Geometry check sheet. Reference: the model listing, model coordinates, mm. Face numbers are marked on the shaded views. Coordinates: 2 decimals unless noted, no trailing zeros. Order: outer loops, then holes, each group sorted by start corner. A loop starts at its lowest first (then second) coordinate and runs counter-clockwise, first axis right, second up. Notation, with made-up numbers: (88.5, 50.25) - (96.5, 50.25) arc R8 cw to (96.5, 57.25) - close; hole circle Ø6 at (-10.5, 69.25). An arc over 180 degrees is marked (long way). Return JSON: item names as keys, results as strings. Group by question number.
Item 1: Section check A-A on y = 0. Enter the section's corners in (x, z).
Item 2: Scan lines: probe 1 along Y at (x, z) = (3.8, 0); probe 2 along Z at (x, y) = (3, 2); probe 3 along Y at (x, z) = (4.75, -1). Record each from-to range of solid material in increasing order.
Item 3: Section check C-C on x = 3. Enter the section's corners in (y, z).
Item 4: Draft check along Z on the marked faces 1 and 2. Enter one of: pulls with the +Z half, pulls with the -Z half, needs draft (parallel to the pull), parting line crosses it, or undercut.
Item 5: Gauge pin test, flat ends, axial feed: pin 1 (4.5 mm diameter, centred on y = 0, z = 39, fed in from -X); pin 2 (1.5 mm diameter, centred on x = 1, z = 14.5, fed in from -Y). Record the tip position at first contact, or that the pin passes through.
Item 6: Section check D-D on y = -11. Enter the section's corners in (x, z).
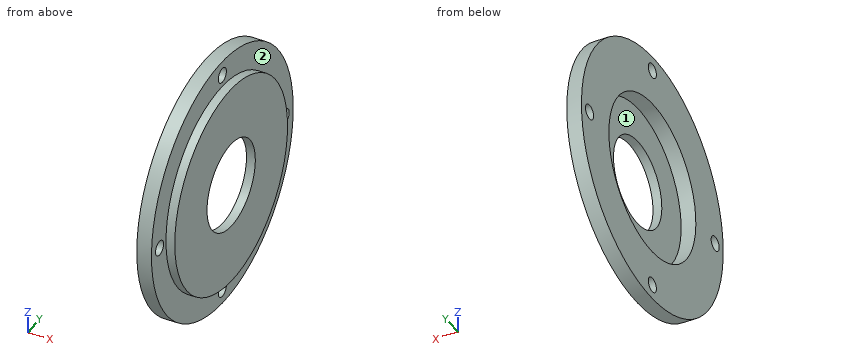
from build123d import *

# Parameters (mm, degrees)
SKETCH_1_R          = 44
SKETCH_1_R_2        = 27
EXTRUDE_1_DEPTH     = 5
SKETCH_2_R          = 35
EXTRUDE_2_DEPTH     = 3
SKETCH_3_R          = 2.5
CUT_EXTRUDE_1_DEPTH = 5
SKETCH_4_R          = 15
CUT_EXTRUDE_2_DEPTH = 8


with BuildPart() as part:
    # 草图1 → 凸台-拉伸1 (new body)
    with BuildSketch(Plane(origin=(0, 0, 0), x_dir=(0, 0, -1), z_dir=(1, 0, 0))):
        Circle(SKETCH_1_R)
        Circle(SKETCH_1_R_2, mode=Mode.SUBTRACT)
    extrude(amount=EXTRUDE_1_DEPTH)

    # 草图2 → 凸台-拉伸2 (add)
    with BuildSketch(Plane(origin=(5, 0, 0), x_dir=(0, 0, -1), z_dir=(1, 0, 0))):
        Circle(SKETCH_2_R)
    extrude(amount=EXTRUDE_2_DEPTH)

    # 草图3 → 切除-拉伸1 (cut)
    with BuildSketch(Plane(origin=(5, 0, 0), x_dir=(0, 0, -1), z_dir=(1, 0, 0))):
        with Locations((0, 39)):
            Circle(SKETCH_3_R)
        with Locations((39, 0)):
            Circle(SKETCH_3_R)
        with Locations((0, -39)):
            Circle(SKETCH_3_R)
        with Locations((-39, 0)):
            Circle(SKETCH_3_R)
    extrude(amount=-CUT_EXTRUDE_1_DEPTH, mode=Mode.SUBTRACT)

    # 草图4 → 切除-拉伸2 (cut)
    with BuildSketch(Plane(origin=(8, 0, 0), x_dir=(0, 0, -1), z_dir=(1, 0, 0))):
        Circle(SKETCH_4_R)
    extrude(amount=-CUT_EXTRUDE_2_DEPTH, mode=Mode.SUBTRACT)


solid = part.part
Computed:
{
 "1": {"outline": "(0, -44) - (5, -44) - (5, -41.5) - (0, -41.5) - close; (0, -36.5) - (5, -36.5) - (5, -35) - (8, -35) - (8, -15) - (5, -15) - (5, -27) - (0, -27) - close; (0, 27) - (5, 27) - (5, 15) - (8, 15) - (8, 35) - (5, 35) - (5, 36.5) - (0, 36.5) - close; (0, 41.5) - (5, 41.5) - (5, 44) - (0, 44) - close"},
 "2": {"probe 1": "y = -44 to -41.5, -36.5 to -27, 27 to 36.5, 41.5 to 44", "probe 2": "z = -43.95 to -40.5, -37.5 to -26.93, 26.93 to 37.5, 40.5 to 43.95", "probe 3": "y = -43.99 to -41.29, -36.71 to -26.98, 26.98 to 36.71, 41.29 to 43.99"},
 "3": {"outline": "circle Ø88 at (0, 0); hole circle Ø5 at (-39, 0); hole circle Ø54 at (0, 0); hole circle Ø5 at (0, -39); hole circle Ø5 at (0, 39); hole circle Ø5 at (39, 0)"},
 "4": {"face 1": "undercut", "face 2": "needs draft"},
 "5": {"pin 1": "passes through", "pin 2": "stops at y = -41.8"},
 "6": {"outline": "(0, -42.6) - (5, -42.6) - (5, -33.23) - (8, -33.23) - (8, -10.2) - (5, -10.2) - (5, -24.66) - (0, -24.66) - close; (0, 24.66) - (5, 24.66) - (5, 10.2) - (8, 10.2) - (8, 33.23) - (5, 33.23) - (5, 42.6) - (0, 42.6) - close"}
}
